Source: CAD feature listing. Evaluate the final solid. Frame: model axes, mm. A direction names the side the tool comes from. Give positions to 0.01 mm unless a question says otherwise; leave off trailing zeros. Write each loop counter-clockwise with the first axis right and the second up, starting at its lowest first coordinate (ties: lowest second). Pieces come first, ordered by that corner, then holes. Notation, with made-up numbers: M 71,12.5 L 102,12.5 A9 ccw 102,22.5 Z; hole C 13,82 d11. An arc over 180 degrees is marked long. Use CSV: the item, a comma, the result in double quotes. Start each with the question number.
from build123d import *

# Parameters (mm, degrees)
CUT_EXTRUDE_1_REACH             = 10
CUT_EXTRUDE_2_REACH             = 36
SKETCH_4_R                      = 1.1
CUT_EXTRUDE_2_DIRECTION_2_REACH = 36


with BuildPart() as part:
    # 草图2 → 旋转1 (revolve)
    with BuildSketch(Plane(origin=(0, 0, 0), x_dir=(1, 0, 0), z_dir=(0, 1, 0))):
        with BuildLine():
            Line((-4, -4), (-4, 4))
            Line((-4, 4), (-34, 4))
            Line((-34, 4), (-34, 2))
            ThreePointArc((-34, 2), (-32, 0), (-34, -2))
            Line((-34, -2), (-34, -4))
            Line((-34, -4), (-7, -4))
            Line((-7, -4), (-7, -14))
            Line((-7, -14), (-4, -14))
            Line((-4, -14), (-4, -4))
        make_face()
    revolve(axis=Axis((0, 0, 0), (0, 0, -1)))

    # 草图3 → 切除-拉伸1 (cut, up to next)
    with BuildSketch(Plane.XY.offset(4), mode=Mode.PRIVATE) as cut_extrude_1_sk1:
        with BuildLine():
            Line((-30, 0), (-8, 0))
            ThreePointArc((-8, 0), (-7.878462024, -1.389185421), (-7.517540966, -2.736161147))
            Line((-7.517540966, -2.736161147), (-28.190778624, -10.2606043))
            ThreePointArc((-28.190778624, -10.2606043), (-29.54423259, -5.20944533), (-30, 0))
        make_face()
    cut_extrude_1_tool1 = extrude(cut_extrude_1_sk1.sketch, amount=-CUT_EXTRUDE_1_REACH, mode=Mode.PRIVATE) & part.part
    add(cut_extrude_1_tool1.solids().sort_by_distance((-20.696454, -3.649343, 4))[0], mode=Mode.SUBTRACT)
    # 草图3 → 切除-拉伸1 (cut, up to next)
    with BuildSketch(Plane.XY.offset(4), mode=Mode.PRIVATE) as cut_extrude_1_sk2:
        with BuildLine():
            Line((-29.54423259, 5.20944533), (-7.878462024, 1.389185421))
            ThreePointArc((-7.878462024, 1.389185421), (-7.517540966, 2.736161147), (-6.92820323, 4))
            Line((-6.92820323, 4), (-25.980762114, 15))
            ThreePointArc((-25.980762114, 15), (-28.190778624, 10.2606043), (-29.54423259, 5.20944533))
        make_face()
    cut_extrude_1_tool2 = extrude(cut_extrude_1_sk2.sketch, amount=-CUT_EXTRUDE_1_REACH, mode=Mode.PRIVATE) & part.part
    add(cut_extrude_1_tool2.solids().sort_by_distance((-19.748327, 7.187803, 4))[0], mode=Mode.SUBTRACT)
    # 草图3 → 切除-拉伸1 (cut, up to next)
    with BuildSketch(Plane.XY.offset(4), mode=Mode.PRIVATE) as cut_extrude_1_sk3:
        with BuildLine():
            Line((-22.981333294, 19.283628291), (-6.128355545, 5.142300877))
            ThreePointArc((-6.128355545, 5.142300877), (-5.142300877, 6.128355545), (-4, 6.92820323))
            Line((-4, 6.92820323), (-15, 25.980762114))
            ThreePointArc((-15, 25.980762114), (-19.283628291, 22.981333294), (-22.981333294, 19.283628291))
        make_face()
    cut_extrude_1_tool3 = extrude(cut_extrude_1_sk3.sketch, amount=-CUT_EXTRUDE_1_REACH, mode=Mode.PRIVATE) & part.part
    add(cut_extrude_1_tool3.solids().sort_by_distance((-13.508651, 16.098984, 4))[0], mode=Mode.SUBTRACT)
    # 草图3 → 切除-拉伸1 (cut, up to next)
    with BuildSketch(Plane.XY.offset(4), mode=Mode.PRIVATE) as cut_extrude_1_sk4:
        with BuildLine():
            Line((-10.2606043, 28.190778624), (-2.736161147, 7.517540966))
            ThreePointArc((-2.736161147, 7.517540966), (-1.389185421, 7.878462024), (0, 8))
            Line((0, 8), (0, 30))
            ThreePointArc((0, 30), (-5.20944533, 29.54423259), (-10.2606043, 28.190778624))
        make_face()
    cut_extrude_1_tool4 = extrude(cut_extrude_1_sk4.sketch, amount=-CUT_EXTRUDE_1_REACH, mode=Mode.PRIVATE) & part.part
    add(cut_extrude_1_tool4.solids().sort_by_distance((-3.649343, 20.696454, 4))[0], mode=Mode.SUBTRACT)
    # 草图3 → 切除-拉伸1 (cut, up to next)
    with BuildSketch(Plane.XY.offset(4), mode=Mode.PRIVATE) as cut_extrude_1_sk5:
        with BuildLine():
            Line((5.20944533, 29.54423259), (1.389185421, 7.878462024))
            ThreePointArc((1.389185421, 7.878462024), (2.736161147, 7.517540966), (4, 6.92820323))
            Line((4, 6.92820323), (15, 25.980762114))
            ThreePointArc((15, 25.980762114), (10.2606043, 28.190778624), (5.20944533, 29.54423259))
        make_face()
    cut_extrude_1_tool5 = extrude(cut_extrude_1_sk5.sketch, amount=-CUT_EXTRUDE_1_REACH, mode=Mode.PRIVATE) & part.part
    add(cut_extrude_1_tool5.solids().sort_by_distance((7.187803, 19.748327, 4))[0], mode=Mode.SUBTRACT)
    # 草图3 → 切除-拉伸1 (cut, up to next)
    with BuildSketch(Plane.XY.offset(4), mode=Mode.PRIVATE) as cut_extrude_1_sk6:
        with BuildLine():
            Line((19.283628291, 22.981333294), (5.142300877, 6.128355545))
            ThreePointArc((5.142300877, 6.128355545), (6.128355545, 5.142300877), (6.92820323, 4))
            Line((6.92820323, 4), (25.980762114, 15))
            ThreePointArc((25.980762114, 15), (22.981333294, 19.283628291), (19.283628291, 22.981333294))
        make_face()
    cut_extrude_1_tool6 = extrude(cut_extrude_1_sk6.sketch, amount=-CUT_EXTRUDE_1_REACH, mode=Mode.PRIVATE) & part.part
    add(cut_extrude_1_tool6.solids().sort_by_distance((16.098984, 13.508651, 4))[0], mode=Mode.SUBTRACT)
    # 草图3 → 切除-拉伸1 (cut, up to next)
    with BuildSketch(Plane.XY.offset(4), mode=Mode.PRIVATE) as cut_extrude_1_sk7:
        with BuildLine():
            Line((28.190778624, 10.2606043), (7.517540966, 2.736161147))
            ThreePointArc((7.517540966, 2.736161147), (7.878462024, 1.389185421), (8, 0))
            Line((8, 0), (30, 0))
            ThreePointArc((30, 0), (29.54423259, 5.20944533), (28.190778624, 10.2606043))
        make_face()
    cut_extrude_1_tool7 = extrude(cut_extrude_1_sk7.sketch, amount=-CUT_EXTRUDE_1_REACH, mode=Mode.PRIVATE) & part.part
    add(cut_extrude_1_tool7.solids().sort_by_distance((20.696454, 3.649343, 4))[0], mode=Mode.SUBTRACT)
    # 草图3 → 切除-拉伸1 (cut, up to next)
    with BuildSketch(Plane.XY.offset(4), mode=Mode.PRIVATE) as cut_extrude_1_sk8:
        with BuildLine():
            Line((29.54423259, -5.20944533), (7.878462024, -1.389185421))
            ThreePointArc((7.878462024, -1.389185421), (7.517540966, -2.736161147), (6.92820323, -4))
            Line((6.92820323, -4), (25.980762114, -15))
            ThreePointArc((25.980762114, -15), (28.190778624, -10.2606043), (29.54423259, -5.20944533))
        make_face()
    cut_extrude_1_tool8 = extrude(cut_extrude_1_sk8.sketch, amount=-CUT_EXTRUDE_1_REACH, mode=Mode.PRIVATE) & part.part
    add(cut_extrude_1_tool8.solids().sort_by_distance((19.748327, -7.187803, 4))[0], mode=Mode.SUBTRACT)
    # 草图3 → 切除-拉伸1 (cut, up to next)
    with BuildSketch(Plane.XY.offset(4), mode=Mode.PRIVATE) as cut_extrude_1_sk9:
        with BuildLine():
            Line((22.981333294, -19.283628291), (6.128355545, -5.142300877))
            ThreePointArc((6.128355545, -5.142300877), (5.142300877, -6.128355545), (4, -6.92820323))
            Line((4, -6.92820323), (15, -25.980762114))
            ThreePointArc((15, -25.980762114), (19.283628291, -22.981333294), (22.981333294, -19.283628291))
        make_face()
    cut_extrude_1_tool9 = extrude(cut_extrude_1_sk9.sketch, amount=-CUT_EXTRUDE_1_REACH, mode=Mode.PRIVATE) & part.part
    add(cut_extrude_1_tool9.solids().sort_by_distance((13.508651, -16.098984, 4))[0], mode=Mode.SUBTRACT)
    # 草图3 → 切除-拉伸1 (cut, up to next)
    with BuildSketch(Plane.XY.offset(4), mode=Mode.PRIVATE) as cut_extrude_1_sk10:
        with BuildLine():
            Line((10.2606043, -28.190778624), (2.736161147, -7.517540966))
            ThreePointArc((2.736161147, -7.517540966), (1.389185421, -7.878462024), (0, -8))
            Line((0, -8), (0, -30))
            ThreePointArc((0, -30), (5.20944533, -29.54423259), (10.2606043, -28.190778624))
        make_face()
    cut_extrude_1_tool10 = extrude(cut_extrude_1_sk10.sketch, amount=-CUT_EXTRUDE_1_REACH, mode=Mode.PRIVATE) & part.part
    add(cut_extrude_1_tool10.solids().sort_by_distance((3.649343, -20.696454, 4))[0], mode=Mode.SUBTRACT)
    # 草图3 → 切除-拉伸1 (cut, up to next)
    with BuildSketch(Plane.XY.offset(4), mode=Mode.PRIVATE) as cut_extrude_1_sk11:
        with BuildLine():
            Line((-5.20944533, -29.54423259), (-1.389185421, -7.878462024))
            ThreePointArc((-1.389185421, -7.878462024), (-2.736161147, -7.517540966), (-4, -6.92820323))
            Line((-4, -6.92820323), (-15, -25.980762114))
            ThreePointArc((-15, -25.980762114), (-10.2606043, -28.190778624), (-5.20944533, -29.54423259))
        make_face()
    cut_extrude_1_tool11 = extrude(cut_extrude_1_sk11.sketch, amount=-CUT_EXTRUDE_1_REACH, mode=Mode.PRIVATE) & part.part
    add(cut_extrude_1_tool11.solids().sort_by_distance((-7.187803, -19.748327, 4))[0], mode=Mode.SUBTRACT)
    # 草图3 → 切除-拉伸1 (cut, up to next)
    with BuildSketch(Plane.XY.offset(4), mode=Mode.PRIVATE) as cut_extrude_1_sk12:
        with BuildLine():
            Line((-19.283628291, -22.981333294), (-5.142300877, -6.128355545))
            ThreePointArc((-5.142300877, -6.128355545), (-6.128355545, -5.142300877), (-6.92820323, -4))
            Line((-6.92820323, -4), (-25.980762114, -15))
            ThreePointArc((-25.980762114, -15), (-22.981333294, -19.283628291), (-19.283628291, -22.981333294))
        make_face()
    cut_extrude_1_tool12 = extrude(cut_extrude_1_sk12.sketch, amount=-CUT_EXTRUDE_1_REACH, mode=Mode.PRIVATE) & part.part
    add(cut_extrude_1_tool12.solids().sort_by_distance((-16.098984, -13.508651, 4))[0], mode=Mode.SUBTRACT)

    # 草图4 → 切除-拉伸2 (cut, up to next)
    with BuildSketch(Plane(origin=(0, 0, 0), x_dir=(0, 0, -1), z_dir=(1, 0, 0)), mode=Mode.PRIVATE) as cut_extrude_2_sk1:
        with Locations((-9, 0)):
            Circle(SKETCH_4_R)
    cut_extrude_2_tool1 = extrude(cut_extrude_2_sk1.sketch, amount=-CUT_EXTRUDE_2_REACH, mode=Mode.PRIVATE) & part.part
    add(cut_extrude_2_tool1.solids().sort_by_distance((0, 0, 9))[0], mode=Mode.SUBTRACT)

    # 草图4 → 切除-拉伸2 direction 2 (cut, up to next)
    with BuildSketch(Plane(origin=(0, 0, 0), x_dir=(0, 0, -1), z_dir=(1, 0, 0)), mode=Mode.PRIVATE) as cut_extrude_2_direction_2_sk1:
        with Locations((-9, 0)):
            Circle(SKETCH_4_R)
    cut_extrude_2_direction_2_tool1 = extrude(cut_extrude_2_direction_2_sk1.sketch, amount=CUT_EXTRUDE_2_DIRECTION_2_REACH, mode=Mode.PRIVATE) & part.part
    add(cut_extrude_2_direction_2_tool1.solids().sort_by_distance((0, 0, 9))[0], mode=Mode.SUBTRACT)


solid = part.part
1. Access query for faces 4 (the cylindrical face through (-6.466, -2.681, 9.07)), 5 (the cylindrical face through (-23.028, -19.227, 0.056)). Directions: +Z, -Z, +X, -X, +Y, -Y. A direction counts if a zero-diameter tool reaches every point of the face in a straight line with its end or side. Return the directions, or none.
2. Section C-C on x = -13. Give the number of separate pieces and of enclosed holes in the cut face, then the cut area to 3 significant figures.
3. First-contact query: pin 1 (6.5 mm diameter, centred on x = -19.5, z = 1, fed in from -Y); pin 2 (3.5 mm diameter, centred on y = 0, z = 9, fed in from +X); pin 3 (5 mm diameter, centred on x = 3.5, y = 16, fed in from +Z). Flat tips, straight axial feed; report the tip coordinate or a pass-through.
4. Section A-A on z = 9. Return loops of the section in (x, y).
5. Pull-direction query (X, two-part tool) for faces 1 (the cylindrical face through (-2.718, -7.524, 0.056)), 2 (the cylindrical face through (-29.53, -5.28, 0.06)), 3 (the cylindrical face through (-18.28, 28.67, -2.99)); classes: released by +X, released by -X, zero draft, split by the parting line, or undercut.
6. Section B-B on z = 5. Return loops of the section in (x, y).
7. Line query: probe 1 along Z at (x, y) = (-4.95, 0); probe 2 along Y at (x, z) = (-11, 2.25); probe 3 along Y at (x, z) = (-14.5, 3.75). Output: solid intervals per line, ascending.
Resolved:
1,face 4,"+Z"
1,face 5,"+Z, -Z"
2,separate pieces,"6"
2,enclosed holes,"0"
2,area,"217 mm2"
3,pin 1,"stops at y = -29.78"
3,pin 2,"stops at x = 7"
3,pin 3,"stops at z = 4"
4,outline,"M -6.91,-1.1 A7 ccw 6.91,-1.1 L 3.85,-1.1 A4 cw -3.85,-1.1 Z; M -6.91,1.1 L -3.85,1.1 A4 cw 3.85,1.1 L 6.91,1.1 A7 ccw Z"
5,face 1,"undercut"
5,face 2,"undercut"
5,face 3,"split by the parting line"
6,outline,"C 0,0 d14; hole C 0,0 d8"
7,probe 1,"z = -4 to 7.9, 10.1 to 14"
7,probe 2,"y = -32.17 to -27.91, -19.05 to -13.11, -6.35 to -4, 0 to 1.94, 6.35 to 9.23, 19.05 to 32.17"
7,probe 3,"y = -30.75 to -26.26, -25.11 to -17.28, -8.37 to -5.28, 0 to 2.56, 8.37 to 12.17, 25.11 to 30.75"
